Read the model definition and answer for the solid it produces. Units are mm, in the model's axes. Face numbers are marked on the shaded views. A direction names the side the tool comes from. Give positions to 0.01 mm unless a question says otherwise; leave off trailing zeros. Write each loop counter-clockwise with the first axis right and the second up, starting at its lowest first coordinate (ties: lowest second). Pieces come first, ordered by that corner, then holes. Notation, with made-up numbers: (72.5, 25) -> (92.5, 25) arc R16 ccw to (92.5, 54) -> close; hole circle Ø6 at (40.25, -37). An arc over 180 degrees is marked (long way). Put each result on its own line as item: value. Start each with the question number.
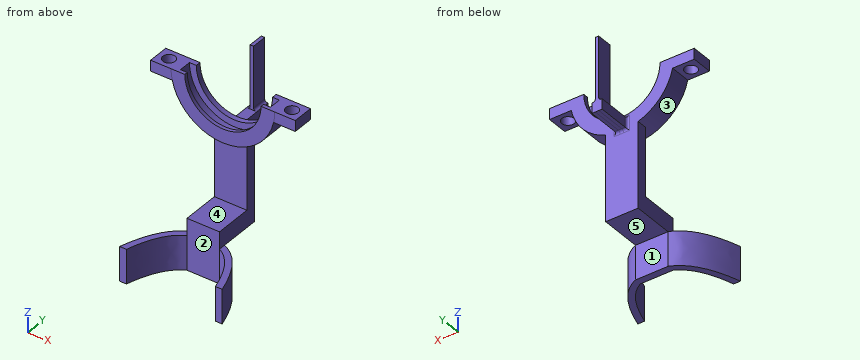
from build123d import *

# Parameters (mm, degrees)
BOSS_EXTRUDE1_DEPTH = 8.5
BOSS_EXTRUDE2_DEPTH = 3
BOSS_EXTRUDE3_DEPTH = 3
SKETCH10_W          = 9.5
SKETCH10_H          = 5
BOSS_EXTRUDE4_DEPTH = 11
SKETCH11_W          = 9.5
SKETCH11_H          = 2
BOSS_EXTRUDE5_DEPTH = 10
BOSS_EXTRUDE6_DEPTH = 6.09393
SKETCH14_R          = 1.8
CUT_EXTRUDE1_DEPTH  = 6.3
SKETCH15_W          = 51.153217575
SKETCH15_H          = 21.210560201
CUT_EXTRUDE3_DEPTH  = 15
SKETCH18_W          = 3
SKETCH18_H          = 3
BOSS_EXTRUDE7_DEPTH = 8.5
FILLET1_R           = 0.75
BOSS_EXTRUDE8_DEPTH = 1.5
FILLET2_R           = 0.75
BOSS_EXTRUDE9_DEPTH = 10


with BuildPart() as part:
    # Sketch3 → Revolve1 (revolve)
    with BuildSketch(Plane.XY):
        Polygon((-62.694264441, 11.733728816), (-64.884531744, 11.733728816), (-64.884531744, 5.639799249), (-60.884531744, 5.639799249), (-60.884531744, 6.650679103), (-62.884531744, 6.650679103), (-62.884531744, 10.250679103), (-60.884531744, 10.250679103), (-60.884531744, 11.733728816), align=None)
    revolve(axis=Axis((-49.744264441, 0, 0), (0, 1, 0)))

    # Sketch7 → Boss-Extrude1 (add)
    with BuildSketch(Plane(origin=(0, 11.733728816, 0), x_dir=(1, 0, 0), z_dir=(0, 1, 0))):
        with BuildLine():
            Line((-50.244264441, 15.132008921), (-50.244264441, 13.130751112))
            ThreePointArc((-50.244264441, 13.130751112), (-49.744264441, 13.140267302), (-49.244264441, 13.130751112))
            Line((-49.244264441, 13.130751112), (-49.244264441, 15.132008921))
            ThreePointArc((-49.244264441, 15.132008921), (-49.744264441, 15.140267302), (-50.244264441, 15.132008921))
        make_face()
    extrude(amount=BOSS_EXTRUDE1_DEPTH)

    # Sketch8 → Boss-Extrude2 (add)
    with BuildSketch(Plane(origin=(0, 20.233728816, 0), x_dir=(1, 0, 0), z_dir=(0, 1, 0))):
        with BuildLine():
            Line((-50.244264441, 15.132008921), (-50.244264441, 13.130751112))
            Line((-50.244264441, 13.130751112), (-50.244264441, -6.369248888))
            Line((-50.244264441, -6.369248888), (-49.244264441, -6.369248888))
            Line((-49.244264441, -6.369248888), (-49.244264441, 13.130751112))
            Line((-49.244264441, 13.130751112), (-49.244264441, 15.132008921))
            ThreePointArc((-49.244264441, 15.132008921), (-49.744264441, 15.140267302), (-50.244264441, 15.132008921))
        make_face()
    extrude(amount=-BOSS_EXTRUDE2_DEPTH)

    # Sketch9 → Boss-Extrude3 (add)
    with BuildSketch(Plane(origin=(0, 11.733728816, 0), x_dir=(1, 0, 0), z_dir=(0, 1, 0))):
        with BuildLine():
            Line((-54.494264441, 14.375854548), (-54.494264441, 39.375854548))
            Line((-54.494264441, 39.375854548), (-44.994264441, 39.375854548))
            Line((-44.994264441, 39.375854548), (-44.994264441, 14.375854548))
            ThreePointArc((-44.994264441, 14.375854548), (-47.092177082, 14.906177465), (-49.244264441, 15.132008921))
            ThreePointArc((-49.244264441, 15.132008921), (-49.744264441, 15.140267302), (-50.244264441, 15.132008921))
            ThreePointArc((-50.244264441, 15.132008921), (-52.3963518, 14.906177465), (-54.494264441, 14.375854548))
        make_face()
    extrude(amount=-BOSS_EXTRUDE3_DEPTH)

    # Sketch10 → Boss-Extrude4 (add)
    with BuildSketch(Plane.XZ.offset(-8.733728816)):
        with Locations((-49.744264441, -36.875854548)):
            Rectangle(SKETCH10_W, SKETCH10_H)
    extrude(amount=BOSS_EXTRUDE4_DEPTH)

    # Sketch11 → Boss-Extrude5 (add)
    with BuildSketch(Plane(origin=(0, 0, -39.375854548), x_dir=(-1, 0, 0), z_dir=(0, 0, -1))):
        with Locations((49.744264441, -1.266271184)):
            Rectangle(SKETCH11_W, SKETCH11_H)
    extrude(amount=BOSS_EXTRUDE5_DEPTH)

    # Sketch13 → Boss-Extrude6 (add)
    with BuildSketch(Plane(origin=(0, 11.733728816, 0), x_dir=(1, 0, 0), z_dir=(0, 1, 0))):
        with BuildLine():
            Line((-28.603997139, 3.15), (-34.935307895, 3.15))
            ThreePointArc((-34.935307895, 3.15), (-34.603997139, 0), (-34.935307895, -3.15))
            Line((-34.935307895, -3.15), (-28.603997139, -3.15))
            Line((-28.603997139, -3.15), (-28.603997139, 3.15))
        make_face()
        with BuildLine():
            Line((-70.884531744, 3.15), (-70.884531744, -3.15))
            Line((-70.884531744, -3.15), (-64.553220987, -3.15))
            ThreePointArc((-64.553220987, -3.15), (-64.884531744, 0), (-64.553220987, 3.15))
            Line((-64.553220987, 3.15), (-70.884531744, 3.15))
        make_face()
    extrude(amount=-BOSS_EXTRUDE6_DEPTH)

    # Sketch14 → Cut-Extrude1 (cut)
    with BuildSketch(Plane.XY.offset(3.15)):
        with Locations((-31.769652517, 8.686764033)):
            Circle(SKETCH14_R)
        with Locations((-67.718876365, 8.686764033)):
            Circle(SKETCH14_R)
    extrude(amount=-CUT_EXTRUDE1_DEPTH, mode=Mode.SUBTRACT)

    # Sketch15 → Cut-Extrude3 (cut, through all)
    with BuildSketch(Plane(origin=(0, 11.733728816, 0), x_dir=(1, 0, 0), z_dir=(0, 1, 0))):
        with Locations((-49.018725857, -10.6052801)):
            Rectangle(SKETCH15_W, SKETCH15_H)
    extrude(amount=-CUT_EXTRUDE3_DEPTH, mode=Mode.SUBTRACT)

    # Sketch18 → Boss-Extrude7 (add)
    with BuildSketch(Plane(origin=(0, 11.733728816, 0), x_dir=(1, 0, 0), z_dir=(0, 1, 0))):
        with Locations((-49.744264441, 13.632008921)):
            Rectangle(SKETCH18_W, SKETCH18_H)
    extrude(amount=BOSS_EXTRUDE7_DEPTH)

    # Fillet1
    fillet1_edges = [part.edges().sort_by_distance(p)[0] for p in [
        (-50.744264441, 11.733728816, -15.132008921),
        (-48.744264441, 11.733728816, -15.132008921),
        (-49.744264441, 11.733728816, -12.132008921),
        (-48.244264441, 11.733728816, -13.632008921),
        (-51.244264441, 11.733728816, -13.632008921),
        (-49.744264441, 11.733728816, -15.140267302),
    ]]
    fillet(fillet1_edges, radius=FILLET1_R)

    # Sketch19 → Boss-Extrude8 (add)
    with BuildSketch(Plane(origin=(0, 20.233728816, 0), x_dir=(1, 0, 0), z_dir=(0, 1, 0))):
        with BuildLine():
            Line((-50.244264441, 15.132008921), (-51.244264441, 15.132008921))
            Line((-51.244264441, 15.132008921), (-51.244264441, 12.132008921))
            Line((-51.244264441, 12.132008921), (-50.244264441, 12.132008921))
            Line((-50.244264441, 12.132008921), (-50.244264441, -6.369248888))
            Line((-50.244264441, -6.369248888), (-49.244264441, -6.369248888))
            Line((-49.244264441, -6.369248888), (-49.244264441, 12.132008921))
            Line((-49.244264441, 12.132008921), (-48.244264441, 12.132008921))
            Line((-48.244264441, 12.132008921), (-48.244264441, 15.132008921))
            Line((-48.244264441, 15.132008921), (-49.244264441, 15.132008921))
            ThreePointArc((-49.244264441, 15.132008921), (-49.744264441, 15.140267302), (-50.244264441, 15.132008921))
        make_face()
    extrude(amount=BOSS_EXTRUDE8_DEPTH)

    # Fillet2
    fillet2_edges = [part.edges().sort_by_distance(p)[0] for p in [
        (-50.244264441, 19.483728816, -12.132008921),
        (-49.244264441, 19.483728816, -12.132008921),
    ]]
    fillet(fillet2_edges, radius=FILLET2_R)

    # Sketch20 → Boss-Extrude9 (add)
    with BuildSketch(Plane(origin=(0, 0, -49.375854548), x_dir=(-1, 0, 0), z_dir=(0, 0, -1))):
        with BuildLine():
            Line((34.744264441, -15.266271184), (36.744264441, -15.266271184))
            add(Edge.make_bspline(
                [(36.744264441, -15.266271184), (39.582311707, -4.870122804), (44.994264441, -2.266271184)],
                knots=[0, 0, 0, 0.599407443, 0.599407443, 0.599407443], degree=2))
            Line((44.994264441, -2.266271184), (54.494264441, -2.266271184))
            add(Edge.make_bspline(
                [(54.494264441, -2.266271184), (59.906217176, -4.870122804), (62.744264441, -15.266271184)],
                knots=[0.400592557, 0.400592557, 0.400592557, 1, 1, 1], degree=2))
            Line((62.744264441, -15.266271184), (64.744264441, -15.266271184))
            add(Edge.make_bspline(
                [(64.744264441, -15.266271184), (61.29176104, -2.966792571), (54.494264441, -0.266271184)],
                knots=[0, 0, 0, 0.639930482, 0.639930482, 0.639930482], degree=2))
            Line((54.494264441, -0.266271184), (44.994264441, -0.266271184))
            add(Edge.make_bspline(
                [(34.744264441, -15.266271184), (38.196767843, -2.966792571), (44.994264441, -0.266271184)],
                knots=[0, 0, 0, 0.639930482, 0.639930482, 0.639930482], degree=2))
        make_face()
    extrude(amount=-BOSS_EXTRUDE9_DEPTH)


solid = part.part
1) For a pull along X with two mould halves and no side action, classify the marked faces 1, 2 and 3 as pulls with the +X half, pulls with the -X half, needs draft (parallel to the pull), parting line crosses it, or undercut.
2) Straight lines are drawn through the part: line 1 (Z direction, x = -53.5, y = 1.5); line 2 (Y direction, x = -53.5, z = -24.5); line 3 (Z direction, x = -48, y = -0.5). For each, find the intervals that lie inside material, in ascending order. Write a range as [from, to].
3) Each of these flat-tipped pins is pushed along its axis until it touches: pin 1 Ø7.5 at (x, z) = (-49, -41) entering from -Y; pin 2 Ø3.5 at (y, z) = (16.5, -14.5) entering from -X; pin 3 Ø1.5 at (x, z) = (-54.5, -22) entering from +Y. Where does it stop, or does it pass through?
4) A cutting plane is placed at C-C on y = 4. Give the vertices of the cut face in (x, z).
5) A cutting plane is placed at B-B on z = 2.5. Give the vertices of the cut face in (x, y), and give its area (3 significant figures).
6) A cutting plane is placed at A-A on x = -32.5. Give the vertices of the cut face in (y, z).
7) For the marked faces 4 and 5, determine the directions among +Z, -Z, +X, -X, +Y, -Y from which every point of the face is accessible in a straight line to the end or side of a thin tool.
Results found:
1. face 1: needs draft
1. face 2: undercut
1. face 3: parting line crosses it
2. line 1: z = [-39.38, -34.38]
2. line 2: y = [8.73, 11.73]
2. line 3: z = [-49.38, -34.38]
3. pin 1: stops at y = -2.27
3. pin 2: stops at x = -51.24
3. pin 3: stops at y = 11.73
4. outline: (-54.49, -39.38) -> (-44.99, -39.38) -> (-44.99, -34.38) -> (-54.49, -34.38) -> close
5. outline: (-50.24, 17.23) -> (-49.24, 17.23) -> (-49.24, 21.73) -> (-50.24, 21.73) -> close
5. area: 4.50 mm²
6. outline: (5.64, -3.15) -> (7.04, -3.15) -> (7.04, 0) -> (5.64, 0) -> close; (10.33, -3.15) -> (11.73, -3.15) -> (11.73, 0) -> (10.33, 0) -> close
7. face 4: +X, -X, -Y
7. face 5: -Z, +X, -X, +Y
